Autodesk Inventor part; units mm, degrees
ref_plane "YZ Plane" through (0, 0, 0) normal (1, 0, 0) x (0, 1, 0)
ref_plane "XZ Plane" through (0, 0, 0) normal (0, 1, 0) x (-1, 0, 0)
ref_plane "XY Plane" through (0, 0, 0) normal (0, 0, 1) x (1, 0, 0)
sketch "Sketch1" plane through (0, 0, 0) normal (0, 0, 1) x (1, 0, 0)
  line L0 (0, 0) -> (72.39, 0)
  line L1 (72.39, 0) -> (72.39, -4.7625)
  line L2 (0, 0) -> (0, -4.7625)
  line L3 (0, -4.7625) -> (72.39, -4.7625)
  circle A0 centre (36.195, -2.3813) radius 2.2098
  dimension "d0" = 72.39
  dimension "d1" = 4.7625
  dimension "d2" = 4.7625
  dimension "d3" = 4.4196
extrude "Extrusion1" add sketch "Sketch1" along normal blind 0.7937
sketch "Sketch2" plane through (0, -4.7625, 0) normal (-1, 0, 0) x (0, 0, 1)
  line L0 (0, 0) -> (0, 4.7625)
  line L1 (0, 4.7625) -> (-179.451, 4.7625)
  line L2 (-179.451, 4.7625) -> (-179.451, 0)
  line L3 (-179.451, 0) -> (0, 0)
  dimension "d6" = 179.451
extrude "Extrusion2" add sketch "Sketch2" against normal blind 0.7937
sketch "Sketch3" plane through (0, -4.7625, -179.451) normal (0, 0, -1) x (-1, 0, 0)
  line L0 (0, 4.7625) -> (0, 0)
  line L1 (-72.39, 0) -> (-72.39, 4.7625)
  line L2 (0, 4.7625) -> (-72.39, 4.7625)
  line L3 (-72.39, 4.7625) -> (-72.39, 0)
  line L4 (-72.39, 0) -> (0, 0)
  line L5 (0, 0) -> (0, 4.7625)
extrude "Extrusion3" add sketch "Sketch3" along normal blind 0.7937
sketch "Sketch4" plane through (72.39, -4.7625, 0) normal (1, 0, 0) x (0, 0, -1)
  line L0 (0, 0) -> (0, 4.7625)
  line L1 (179.451, 4.7625) -> (0, 4.7625)
  line L2 (0, 4.7625) -> (179.451, 4.7625)
  line L3 (0, 0) -> (179.451, 0)
  line L4 (179.451, 4.7625) -> (179.451, 0)
  line L5 (179.451, 0) -> (0, 0)
  line L6 (0, 0) -> (0, 4.7625)
extrude "Extrusion4" add sketch "Sketch4" against normal blind 0.7937
pattern_circular "Circular Pattern1" count 12 over 360 about axis through (36.195, -2.3813, 0) along (0, 0, 1) of "Extrusion3", "Extrusion2", "Extrusion1", "Extrusion4"
properties part number "Rubber Band"
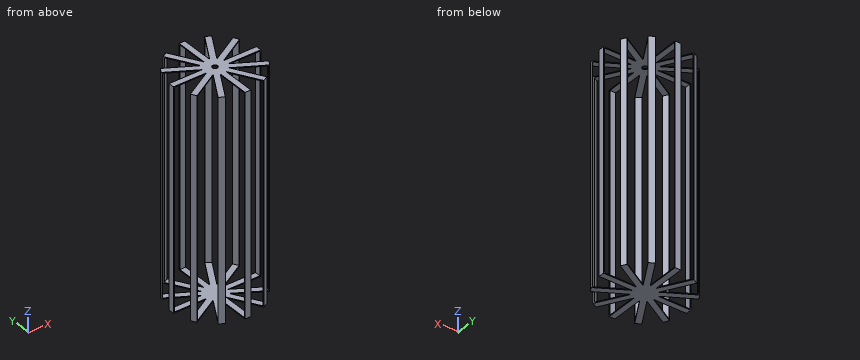
Source: CAD feature listing. Evaluate the final solid. Frame: model axes, mm. Coordinates: 2 decimals unless noted, no trailing zeros. Order: outer loops, then holes, each group sorted by start corner. A loop starts at its lowest first (then second) coordinate and runs counter-clockwise, first axis right, second up. Notation, with made-up numbers: (-20.75, 84.25) - (30.25, 84.25) arc R20 ccw to (30.25, 92.25) - close; hole circle Ø8 at (-9.75, 75). An arc over 180 degrees is marked (long way). One line per item, written item: value.
1) Contact query for flat-ended pins moving along their axis: pin 1 (1 mm diameter, centred on x = 31.5, z = -32.5, fed in from +Y); pin 2 (3 mm diameter, centred on x = 19, z = -112.5, fed in from -Y); pin 3 (8 mm diameter, centred on x = 59, z = -100.5, fed in from -Y); pin 4 (13.5 mm diameter, centred on y = 20.5, z = -92, fed in from -X). Output: stop coordinate, or through.
Computed values:
pin 1: passes through
pin 2: stops at y = -34.92
pin 3: stops at y = -33.32
pin 4: stops at x = 3.71
2) Cut plane C-C on z = -59.5. State how many separate pieces and enclosed holes the cut face has, plus the area to 3 significant figures.
Computed values:
separate pieces: 12
enclosed holes: 0
area: 45.4 mm^2
3) Cut plane B-B on x = 60. Output: boundary loops of the cut face in (y, z).
Computed values:
outline: (-18.87, -180.24) - (-13.38, -180.24) - (-13.38, -179.45) - (-18.87, -179.45) - close; (-18.87, 0) - (-13.38, 0) - (-13.38, 0.79) - (-18.87, 0.79) - close; (-4.76, -180.24) - (0, -180.24) - (0, -179.45) - (-4.76, -179.45) - close; (-4.76, 0) - (0, 0) - (0, 0.79) - (-4.76, 0.79) - close; (8.61, -180.24) - (14.11, -180.24) - (14.11, -179.45) - (8.61, -179.45) - close; (8.61, 0) - (14.11, 0) - (14.11, 0.79) - (8.61, 0.79) - close
4) Ray query, line 1 (Z direction, x = 52.5, y = -26); line 2 (Y direction, x = 37, z = -102); line 3 (Y direction, x = 20, z = -29.5). Return the intervals inside material, ascending. Write a range as [from, to].
Computed values:
line 1: z = [-180.24, -179.45], [0, 0.79]
line 2: y = [-38.58, -37.78], [33.02, 33.81]
line 3: y = [-34.83, -33.91], [29.15, 30.06]
5) Cut plane A-A on y = 23.5. Output: boundary loops of the cut face in (x, z).
Computed values:
outline: (18.5, -180.24) - (24, -180.24) - (24, -179.45) - (18.5, -179.45) - close; (18.5, 0) - (24, 0) - (24, 0.79) - (18.5, 0.79) - close; (33.81, -180.24) - (38.58, -180.24) - (38.58, -179.45) - (33.81, -179.45) - close; (33.81, 0) - (38.58, 0) - (38.58, 0.79) - (33.81, 0.79) - close; (48.39, -180.24) - (53.89, -180.24) - (53.89, -179.45) - (48.39, -179.45) - close; (48.39, 0) - (53.89, 0) - (53.89, 0.79) - (48.39, 0.79) - close
